```python
from build123d import *

# Parameters (mm, degrees)
F0_R     = 76
F1_DEPTH = 10
F2_R     = 4
F3_DEPTH = 10
F4_DEPTH = 250
F5_R     = 70
F6_DEPTH = 250


with BuildPart() as f1:
    # F0 (on Top) → F1 (new body)
    with BuildSketch(Plane.XY):
        Circle(F0_R)
    extrude(amount=F1_DEPTH)

    # F2 (on face) → F3 (cut, through all)
    with BuildSketch(Plane.XY.offset(10)):
        with Locations((-60, 0)):
            Circle(F2_R)
        with Locations((60, 0)):
            Circle(F2_R)
        with Locations((0, -60)):
            Circle(F2_R)
        with Locations((0, 60)):
            Circle(F2_R)
    extrude(amount=-F3_DEPTH, mode=Mode.SUBTRACT)

    # F4 (add): a face of the model
    f4_faces = [f1.faces().sort_by_distance(p)[0] for p in [
        (0, 0, 0),
    ]]
    extrude(f4_faces, amount=F4_DEPTH)

    # F5 (on face) → F6 (cut, through all)
    with BuildSketch(Plane(origin=(0, 0, -250), x_dir=(1, 0, 0), z_dir=(0, 0, -1))):
        Circle(F5_R)
    extrude(amount=-F6_DEPTH, mode=Mode.SUBTRACT)


solid = f1.part
```
CAD build for the part. Positions are in the model's coordinates, mm. A direction names the side the tool comes from. Coordinates: 2 decimals unless noted, no trailing zeros. Order: outer loops, then holes, each group sorted by start corner. A loop starts at its lowest first (then second) coordinate and runs counter-clockwise, first axis right, second up. Notation, with made-up numbers: (22.25, 46) - (81.25, 46) arc R20 ccw to (81.25, 51) - close; hole circle Ø1 at (6, 89). An arc over 180 degrees is marked (long way). Answer in a Markdown table with one row per item.
1. Slice it at D-D, the plane x = -48. List the corners of the cut face in (y, z).
Answer:
| item | result |
|---|---|
| outline | (-58.92, -250) - (-50.95, -250) - (-50.95, 0) - (50.95, 0) - (50.95, -250) - (58.92, -250) - (58.92, 10) - (-58.92, 10) - close |
2. Flat gauge pins, fed straight in: P1, Ø10.5, axis at x = 60, y = 0, coming from the -Z side; P2, Ø7, axis at x = -60, y = 0, coming from the -Z side; P3, Ø12, axis at x = 25, z = -197, coming from the -Y side; P4, Ø1, axis at x = 0.5, z = -73.5, coming from the -Y side. Where does each tip first touch, or does it go through?
Answer:
| item | result |
|---|---|
| P1 | z = 0 |
| P2 | through |
| P3 | y = -73.59 |
| P4 | y = -76 |
3. Drill centre lines: L1, parallel to Y at x = 0, z = 6.75; L2, parallel to Z at x = 31, y = 52.5; L3, parallel to X at y = -3.5, z = -213. Where is each one in solid material? Low to high. Write a range as from..to.
Answer:
| item | result |
|---|---|
| L1 | -76..-64, -56..56, 64..76 |
| L2 | 0..10 |
| L3 | -75.92..-69.91, 69.91..75.92 |
4. Slice it at B-B, the plane x = 60. List the corners of the cut face in (y, z), then the cut area to 3 significant figures.
Answer:
| item | result |
|---|---|
| outline | (-46.65, -250) - (-36.06, -250) - (-36.06, 0) - (-4, 0) - (-4, 10) - (-46.65, 10) - close; (4, 0) - (36.06, 0) - (36.06, -250) - (46.65, -250) - (46.65, 10) - (4, 10) - close |
| area | 6,150 mm² |
5. Pull direction X, two halves, no side cores. Call faces 3 (the face through (35.069, -67.425, -118.18)), 4 (the face through (-0.867, 56.095, 5.07)), 5 (the face through (33, -62, -250)): +X half, -X half, draft (parallel to the pull), parting line (faces both ways), or undercut.
Answer:
| item | result |
|---|---|
| face 3 | parting line |
| face 4 | undercut |
| face 5 | draft |
6. Slice it at A-A, the plane y = 0. List the corners of the cut face in (x, z).
Answer:
| item | result |
|---|---|
| outline | (-76, -250) - (-70, -250) - (-70, 0) - (-64, 0) - (-64, 10) - (-76, 10) - close; (-56, 0) - (56, 0) - (56, 10) - (-56, 10) - close; (64, 0) - (70, 0) - (70, -250) - (76, -250) - (76, 10) - (64, 10) - close |
7. 3-axis set-ups, long thin cutter, end or side, ignore diameter. For faces 1 (the face through (-1, -1, 0)), 2 (the face through (-0.867, -63.905, 5.07)): which of +Z, -Z, +X, -X, +Y, -Y reach the whole face in a straight line?
Answer:
| item | result |
|---|---|
| face 1 | -Z |
| face 2 | +Z, -Z |
